from build123d import *

# Parameters (mm, degrees)
SKETCH2_W           = 23.75
SKETCH2_H           = 32
BOSS_EXTRUDE1_DEPTH = 5
SKETCH3_W           = 23.75
SKETCH3_H           = 40
BOSS_EXTRUDE2_DEPTH = 5
BOSS_EXTRUDE3_START = -11.875
BOSS_EXTRUDE3_DEPTH = 9
SKETCH5_R           = 7.5
SKETCH5_R_2         = 5
BOSS_EXTRUDE4_DEPTH = 12
BOSS_EXTRUDE4_DRAFT = 5
SKETCH6_R           = 5
BOSS_EXTRUDE5_DEPTH = 5
BOSS_EXTRUDE5_TAPER = 45
FILLET1_R           = 2


with BuildPart() as part:
    # Sketch2 → Boss-Extrude1 (new body)
    with BuildSketch(Plane.XY):
        Rectangle(SKETCH2_W, SKETCH2_H)
    extrude(amount=-BOSS_EXTRUDE1_DEPTH)

    # Sketch3 → Boss-Extrude2 (add)
    with BuildSketch(Plane.XY):
        with Locations((0, 4)):
            Rectangle(SKETCH3_W, SKETCH3_H)
    extrude(amount=BOSS_EXTRUDE2_DEPTH)

    # Sketch4 → Boss-Extrude3 (add, symmetric)
    with BuildSketch(Plane(origin=(11.875, 0, 0), x_dir=(0, 0, -1), z_dir=(1, 0, 0)).offset(BOSS_EXTRUDE3_START)):
        Polygon((-5, -3.277778494), (-15, 14.042729581), (-20.629165125, 10.792729581), (-5, -16), align=None)
    extrude(amount=BOSS_EXTRUDE3_DEPTH, both=True)


with BuildPart() as boss_extrude4_tool:
    # Sketch5 → Boss-Extrude4 (with draft: the straight prism first)
    with BuildSketch(Plane(origin=(0, -6.238375225, 10.694307668), x_dir=(1, 0, 0), z_dir=(0, -0.50387277832175, 0.863777878430746))):
        Circle(SKETCH5_R)
        Circle(SKETCH5_R_2, mode=Mode.SUBTRACT)
    extrude(amount=BOSS_EXTRUDE4_DEPTH)
    # Boss-Extrude4: the draft: its side faces are tilted about the plane it starts from
    boss_extrude4_sides = [boss_extrude4_tool.faces().sort_by_distance(p)[0] for p in [
        (-7.5, -9.261611895, 15.876974938),
        (-5, -9.261611895, 15.876974938),
    ]]
    draft(boss_extrude4_sides, Plane(origin=(0, -6.238375225, 10.694307668), x_dir=(1, 0, 0), z_dir=(0, -0.50387277832175, 0.863777878430746)), BOSS_EXTRUDE4_DRAFT)


with BuildPart() as part_1:
    add(part.part)

    # Boss-Extrude4: add boss_extrude4_tool
    add(boss_extrude4_tool.part)

    # Sketch6 → Boss-Extrude5 (add)
    with BuildSketch(Plane(origin=(0, -6.238375225, 10.694307668), x_dir=(1, 0, 0), z_dir=(0, -0.50387277832175, 0.863777878430746))):
        Circle(SKETCH6_R)
    extrude(amount=BOSS_EXTRUDE5_DEPTH, taper=BOSS_EXTRUDE5_TAPER)

    # Fillet1
    fillet1_edges = [part_1.edges().sort_by_distance(p)[0] for p in [
        (-11.875, 24, 2.5),
        (11.875, 24, 2.5),
        (0, -3.277778494, 5),
        (-9, 12.417729581, 17.814582562),
        (9, 12.417729581, 17.814582562),
    ]]
    fillet(fillet1_edges, radius=FILLET1_R)


solid = part_1.part
Source: CAD feature listing. Evaluate the final solid. Frame: model axes, mm. A direction names the side the tool comes from. Round coordinates to 2 decimals unless told otherwise and drop trailing zeros. Order: outer loops, then holes, each group sorted by start corner. A loop starts at its lowest first (then second) coordinate and runs counter-clockwise, first axis right, second up. Notation, with made-up numbers: (-4, -9) - (5, -9) arc R32 ccw to (5, 26) - close; hole circle Ø6 at (64, 56). An arc over 180 degrees is marked (long way). Use a Markdown table: item, result. Add a question column.
1. Section query B-B (z = -1). Return the cut outline in (x, y) (3 decimals), then the cut area to 3 significant figures.
2. Mould query, pull axis Z, two halves, no side actions, for faces 1 (the cylindrical face through (-8, 12, 18)), 2 (the conical face through (-4.379, -12.119, 14.113)), 3 (the flat face through (11.875, 3, 0)). Classes: +Z half, -Z half, draft (parallel to the pull), parting line (faces both ways), or undercut.
3. Set-up query: faces 4 (the flat face through (0, 20, 0)), 5 (the flat face through (-9, -2, 11)), 6 (the conical face through (-0.293, -9.217, 13.178)). Return all of +Z, -Z, +X, -X, +Y, -Y with unobstructed straight access to the full face (end or side cutting, diameter ignored); none if empty.
4. Section query A-A (y = 20). Return the cut outline in (x, z) (3 decimals), then the cut area to 3 significant figures.
5. Line query: probe 1 along X at (y, z) = (-3.5, 13); probe 2 along Y at (x, z) = (2.5, 3.5); probe 3 along Y at (x, z) = (7.75, -0.75). Output: solid intervals per line, ascending.
6. First-contact query: pin 1 (2 mm diameter, centred on x = -6, y = 16.5, fed in from +Z); pin 2 (11.5 mm diameter, centred on y = -0.5, z = 14, fed in from +X); pin 3 (4.5 mm diameter, centred on y = -1.5, z = 13.5, fed in from -X); pin 4 (3 mm diameter, centred on y = 19.5, z = 8, fed in from -X). Flat tips, straight axial feed; report the tip coordinate or a pass-through.
Derived:
| question | item | result |
|---|---|---|
| 1 | outline | (-11.875, -16) - (11.875, -16) - (11.875, 16) - (-11.875, 16) - close |
| 1 | area | 760 mm2 |
| 2 | face 1 | +Z half |
| 2 | face 2 | undercut |
| 2 | face 3 | draft |
| 3 | face 4 | -Z, +X, -X, +Y |
| 3 | face 5 | +Z, -X, +Y, -Y |
| 3 | face 6 | none |
| 4 | outline | (-11.875, 0) - (11.875, 0) - (11.875, 5) - (-11.875, 5) - close |
| 4 | area | 119 mm2 |
| 5 | probe 1 | -6.56 to -3.62, -2.61 to 2.61, 3.62 to 6.56 |
| 5 | probe 2 | -16 to 24 |
| 5 | probe 3 | -16 to 16 |
| 6 | pin 1 | z = 5 |
| 6 | pin 2 | x = 9 |
| 6 | pin 3 | x = -9 |
| 6 | pin 4 | through |
